Could you check a few things on this model? Use its own coordinates, in mm. Face numbers are marked on the shaded views. A direction names the side the tool comes from. Round coordinates to 2 decimals unless told otherwise and drop trailing zeros. Order: outer loops, then holes, each group sorted by start corner. A loop starts at its lowest first (then second) coordinate and runs counter-clockwise, first axis right, second up. Notation, with made-up numbers: (66, 65.25) - (93, 65.25) arc R10 cw to (93, 74.25) - close; hole circle Ø9 at (89, 47). An arc over 180 degrees is marked (long way). Return JSON: item names as keys, results as strings. Group by question number.
from build123d import *

# Parameters (mm, degrees)
CUT_EXTRUDE1_DEPTH      = 37.935755035
CUT_EXTRUDE1_DEPTH_BACK = 37.935755035
SKETCH2_R               = 2
FILLET1_R               = 1.5


with BuildPart() as part:
    # Sketch1 → Revolve1 (revolve)
    with BuildSketch(Plane.XY, mode=Mode.PRIVATE) as revolve1_sk:
        Polygon((0, 3.5), (16, 3.5), (16, 1), (26, 1), (26, -2.5), (15, -2.5), (15, -3.5), (0, -3.5), align=None)
    revolve(revolve1_sk.sketch.rotate(Axis((0, 3.5, 0), (0, -1, 0)), 90), axis=Axis((0, 3.5, 0), (0, -1, 0)))

    # Sketch2 → Cut-Extrude1 (cut, two sides: drawn at the far end of the back side and taken through both)
    with BuildSketch(Plane(origin=(0, 0, 0), x_dir=(1, 0, 0), z_dir=(0, 1, 0)).offset(-CUT_EXTRUDE1_DEPTH_BACK)):
        with Locations(Location((-21.5, 0, 0), (0, 0, 270))):
            Circle(SKETCH2_R)
        with Locations(Location((-10.75, -18.619546181, 0), (0, 0, 270))):
            Circle(SKETCH2_R)
        with Locations(Location((10.75, -18.619546181, 0), (0, 0, 270))):
            Circle(SKETCH2_R)
        with Locations(Location((21.5, 0, 0), (0, 0, 270))):
            Circle(SKETCH2_R)
        with Locations(Location((10.75, 18.619546181, 0), (0, 0, 270))):
            Circle(SKETCH2_R)
        with Locations(Location((-10.75, 18.619546181, 0), (0, 0, 270))):
            Circle(SKETCH2_R)
    extrude(amount=CUT_EXTRUDE1_DEPTH + CUT_EXTRUDE1_DEPTH_BACK, mode=Mode.SUBTRACT)

    # Fillet1
    fillet1_edges = [part.edges().sort_by_distance(p)[0] for p in [
        (0, 3.5, -16),
    ]]
    fillet(fillet1_edges, radius=FILLET1_R)


solid = part.part
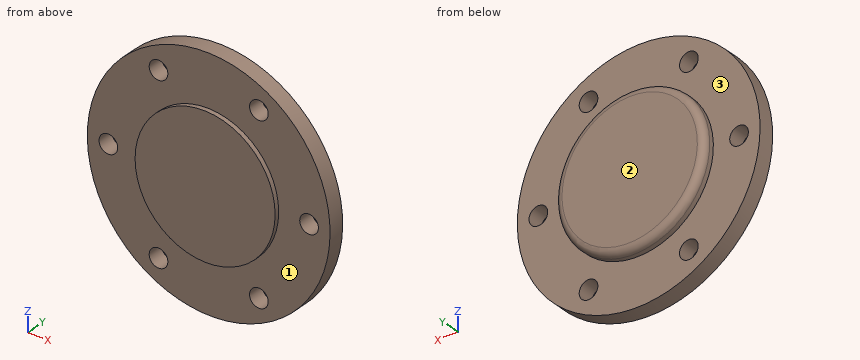
1) Will these pins go through, and if not, where does the flat tip stop? pin 1 (4.5 mm diameter, centred on x = 21.5, z = 0, fed in from +Y); pin 2 (3 mm diameter, centred on x = -10.75, z = -18.62, fed in from +Y); pin 3 (2 mm diameter, centred on y = -2, z = 8.5, fed in from +X); pin 4 (3 mm diameter, centred on y = -2, z = 0, fed in from +X).
2) I want a section at C-C, the plane y = -1.25. List the corners of the cut face in (x, z) for me.
3) I want a section at D-D, the plane x = 0. List the corners of the cut face in (y, z) for me, plus the area to 3 significant figures.
4) If I drill on line 1 along X through (y, z) = (-1.1, 0); line 2 along X through (y, z) = (0.25, 17); line 3 along Z through (x, y) = (-10.75, -1.15), over which ranges is the centre line in solid material (lowest first)? Write a range as from..to.
5) I want a section at B-B, the plane x = 21.5. List the corners of the cut face in (y, z) for me.
6) I want a section at A-A, the plane z = 0. List the corners of the cut face in (x, y) for me, plus the area to 3 significant figures.
7) For the marked faces 1, 2 and 3, which set-ups out of +Z, -Z, +X, -X, +Y, -Y let a thin tool reach every point of the face, with its end or its side?
Outcome:
{
 "1": {"pin 1": "y = 1", "pin 2": "through", "pin 3": "x = 24.89", "pin 4": "x = 26"},
 "2": {"outline": "circle Ø52 at (0, 0); hole circle Ø4 at (-21.5, 0); hole circle Ø4 at (-10.75, -18.62); hole circle Ø4 at (-10.75, 18.62); hole circle Ø4 at (10.75, -18.62); hole circle Ø4 at (10.75, 18.62); hole circle Ø4 at (21.5, 0)"},
 "3": {"outline": "(-3.5, -15) - (-2.5, -15) - (-2.5, -26) - (1, -26) - (1, -16) - (2, -16) arc R1.5 ccw to (3.5, -14.5) - (3.5, 14.5) arc R1.5 ccw to (2, 16) - (1, 16) - (1, 26) - (-2.5, 26) - (-2.5, 15) - (-3.5, 15) - close", "area": "291 mm^2"},
 "4": {"line 1": "-26..-23.5, -19.5..19.5, 23.5..26", "line 2": "-19.67..-11.92, -9.58..9.58, 11.92..19.67", "line 3": "-23.67..-20.62, -16.62..16.62, 20.62..23.67"},
 "5": {"outline": "(-2.5, -14.62) - (1, -14.62) - (1, -2) - (-2.5, -2) - close; (-2.5, 2) - (1, 2) - (1, 14.62) - (-2.5, 14.62) - close"},
 "6": {"outline": "(-26, -2.5) - (-23.5, -2.5) - (-23.5, 1) - (-26, 1) - close; (-19.5, -2.5) - (-15, -2.5) - (-15, -3.5) - (15, -3.5) - (15, -2.5) - (19.5, -2.5) - (19.5, 1) - (16, 1) - (16, 2) arc R1.5 ccw to (14.5, 3.5) - (-14.5, 3.5) arc R1.5 ccw to (-16, 2) - (-16, 1) - (-19.5, 1) - close; (23.5, -2.5) - (26, -2.5) - (26, 1) - (23.5, 1) - close", "area": "263 mm^2"},
 "7": {"face 1": "-Y", "face 2": "+Z, -Z, +X, -X, +Y", "face 3": "+Y"}
}
